The listing builds one solid part. Answer for the finished solid, in the listing's coordinates (mm). Face numbers are marked on the shaded views. A direction names the side the tool comes from. Round coordinates to 2 decimals unless told otherwise and drop trailing zeros. Write each loop counter-clockwise with the first axis right and the second up, starting at its lowest first coordinate (ties: lowest second). Pieces come first, ordered by that corner, then holes. Notation, with made-up numbers: (-3, -18.5) - (34, -18.5) arc R32 ccw to (34, 12.5) - close; hole circle Ø6 at (82.5, 87.25). An arc over 180 degrees is marked (long way). Answer in a Markdown table with one row per item.
from build123d import *

# Parameters (mm, degrees)
SKETCH1_W          = 203.2
SKETCH1_H          = 152.4
BASE_EXTRUDE_DEPTH = 63.5
CUT_EXTRUDE1_DEPTH = 50.8


with BuildPart() as part:
    # Sketch1 → Base-Extrude (new body)
    with BuildSketch(Plane.XY):
        Rectangle(SKETCH1_W, SKETCH1_H)
    extrude(amount=-BASE_EXTRUDE_DEPTH)

    # Sketch2 → Cut-Extrude1 (cut)
    with BuildSketch(Plane.XY):
        with BuildLine():
            Line((-69.85, 57.15), (-25.4, 57.15))
            ThreePointArc((-25.4, 57.15), (-16.419743879, 53.430256121), (-12.7, 44.45))
            Line((-12.7, 44.45), (-12.7, -44.45))
            ThreePointArc((-12.7, -44.45), (-16.419743879, -53.430256121), (-25.4, -57.15))
            Line((-25.4, -57.15), (-69.85, -57.15))
            ThreePointArc((-69.85, -57.15), (-78.830256121, -53.430256121), (-82.55, -44.45))
            Line((-82.55, -44.45), (-82.55, 44.45))
            ThreePointArc((-82.55, 44.45), (-78.830256121, 53.430256121), (-69.85, 57.15))
        make_face()
        with BuildLine():
            Line((19.05, 57.15), (63.5, 57.15))
            ThreePointArc((63.5, 57.15), (72.480256121, 53.430256121), (76.2, 44.45))
            Line((76.2, 44.45), (76.2, -44.45))
            ThreePointArc((76.2, -44.45), (72.480256121, -53.430256121), (63.5, -57.15))
            Line((63.5, -57.15), (19.05, -57.15))
            ThreePointArc((19.05, -57.15), (10.069743879, -53.430256121), (6.35, -44.45))
            Line((6.35, -44.45), (6.35, 44.45))
            ThreePointArc((6.35, 44.45), (10.069743879, 53.430256121), (19.05, 57.15))
        make_face()
    extrude(amount=-CUT_EXTRUDE1_DEPTH, mode=Mode.SUBTRACT)


solid = part.part
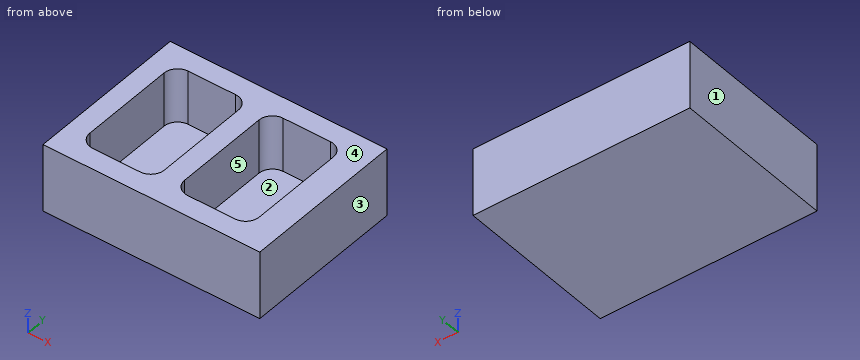
(1) Section D-D (y = 50) is taken. Give the vertices of the cut face in (x, z), and give its area (3 significant figures).
Checked values:
| item | result |
|---|---|
| outline | (-101.6, -63.5) - (101.6, -63.5) - (101.6, 0) - (74.92, 0) - (74.92, -50.8) - (7.63, -50.8) - (7.63, 0) - (-13.98, 0) - (-13.98, -50.8) - (-81.27, -50.8) - (-81.27, 0) - (-101.6, 0) - close |
| area | 6,070 mm2 |
(2) Section C-C (x = 55) is taken. Give the vertices of the cut face in (y, z), and give its area (3 significant figures).
Checked values:
| item | result |
|---|---|
| outline | (-76.2, -63.5) - (76.2, -63.5) - (76.2, 0) - (57.15, 0) - (57.15, -50.8) - (-57.15, -50.8) - (-57.15, 0) - (-76.2, 0) - close |
| area | 3,870 mm2 |
(3) For a pull along X with two mould halves and no side action, classify the marked faces 1, 2 and 3 as pulls with the +X half, pulls with the -X half, needs draft (parallel to the pull), parting line crosses it, or undercut.
Checked values:
| item | result |
|---|---|
| face 1 | pulls with the -X half |
| face 2 | undercut |
| face 3 | pulls with the +X half |
(4) For the marked faces 4 and 5, determine the directions among +Z, -Z, +X, -X, +Y, -Y from which every point of the face is accessible in a straight line to the end or side of a thin tool.
Checked values:
| item | result |
|---|---|
| face 4 | +Z, +X, -X, +Y, -Y |
| face 5 | +Z |
(5) Find the intervals of material crossed by line 1 (X direction, y = -18, z = -37.5); line 2 (Y direction, x = -26, z = -15); line 3 (Z direction, x = -37.5, y = -43.5), in increasing order.
Checked values:
| item | result |
|---|---|
| line 1 | x = -101.6 to -82.55, -12.7 to 6.35, 76.2 to 101.6 |
| line 2 | y = -76.2 to -57.15, 57.15 to 76.2 |
| line 3 | z = -63.5 to -50.8 |
(6) Section A-A (z = -26.5) is taken. Give the vertices of the cut face in (x, y), and give its area (3 significant figures).
Checked values:
| item | result |
|---|---|
| outline | (-101.6, -76.2) - (101.6, -76.2) - (101.6, 76.2) - (-101.6, 76.2) - close; hole (-82.55, -44.45) arc R12.7 ccw to (-69.85, -57.15) - (-25.4, -57.15) arc R12.7 ccw to (-12.7, -44.45) - (-12.7, 44.45) arc R12.7 ccw to (-25.4, 57.15) - (-69.85, 57.15) arc R12.7 ccw to (-82.55, 44.45) - close; hole (6.35, -44.45) arc R12.7 ccw to (19.05, -57.15) - (63.5, -57.15) arc R12.7 ccw to (76.2, -44.45) - (76.2, 44.45) arc R12.7 ccw to (63.5, 57.15) - (19.05, 57.15) arc R12.7 ccw to (6.35, 44.45) - close |
| area | 15,300 mm2 |
(7) Section B-B (y = 15) is taken. Give the vertices of the cut face in (x, z).
Checked values:
| item | result |
|---|---|
| outline | (-101.6, -63.5) - (101.6, -63.5) - (101.6, 0) - (76.2, 0) - (76.2, -50.8) - (6.35, -50.8) - (6.35, 0) - (-12.7, 0) - (-12.7, -50.8) - (-82.55, -50.8) - (-82.55, 0) - (-101.6, 0) - close |
(8) A flat-ended cylindrical pin translates along its axis: pin 1 (2 mm diameter, centred on x = -40, y = 16.5, fed in from +Z). Find the tip coordinate at first contact, or state that the pin passes through.
Checked values:
| item | result |
|---|---|
| pin 1 | stops at z = -50.8 |
